from build123d import *

# Parameters (mm, degrees)
CROQUIS1_R                   = 3
CROQUIS1_R_2                 = 2
SALIENTE_EXTRUIR1_DEPTH      = 3.9
SALIENTE_EXTRUIR2_DEPTH      = 3.9
SALIENTE_EXTRUIR2_DEPTH_BACK = 3.9
REDONDEO1_R                  = 5
CROQUIS4_W                   = 2
CROQUIS4_H                   = 2
CORTAR_EXTRUIR1_DEPTH        = 46.769422107
CROQUIS5_R                   = 3.25
CORTAR_EXTRUIR2_DEPTH        = 46.769422107
REDONDEO3_R                  = 1


with BuildPart() as part:
    # Croquis1 → Saliente-Extruir1 (new body)
    with BuildSketch(Plane(origin=(0, 0, 0), x_dir=(1, 0, 0), z_dir=(0, 1, 0))):
        with Locations(Location((0, 0, 0), (0, 0, 270))):
            Circle(CROQUIS1_R)
        with Locations(Location((0, 0, 0), (0, 0, 270))):
            Circle(CROQUIS1_R_2, mode=Mode.SUBTRACT)
    extrude(amount=SALIENTE_EXTRUIR1_DEPTH)

    # Croquis3 → Saliente-Extruir2 (add, two sides: drawn at the far end of the back side and taken through both)
    with BuildSketch(Plane.XZ.offset(-SALIENTE_EXTRUIR2_DEPTH_BACK)):
        with BuildLine():
            Line((45, 3), (0, 3))
            ThreePointArc((0, 3), (2.121320344, 2.121320344), (3, 0))
            Line((3, 0), (45, 0))
            Line((45, 0), (45, 3))
        make_face()
    extrude(amount=SALIENTE_EXTRUIR2_DEPTH + SALIENTE_EXTRUIR2_DEPTH_BACK)

    # Redondeo1
    # the kernel refuses this fillet: 5 mm, written as the material it takes off along each edge
    with BuildSketch(Plane(origin=(45, 15.356439237, 0), x_dir=(-1, 0, 0), z_dir=(0, -1, 0))) as redondeo1_piece_1:
        with BuildLine():
            CenterArc((4.582575695, -5), REDONDEO1_R, 90, 66.421821522)
            Line((0, -3), (-0.091651514, -2.96))
            ThreePointArc((-0.091651514, -2.96), (-0.1, -1.5), (-0.1, 0))
            Line((-0.1, 0), (0, 0.1))
            Line((0, 0.1), (4.582575695, 0.1))
            Line((4.582575695, 0.1), (4.582575695, 0))
        make_face()
    extrude(amount=30.712878475, mode=Mode.SUBTRACT)

    # Croquis4 → Cortar-Extruir1 (cut, through all)
    with BuildSketch(Plane.XZ.offset(3.9)):
        with Locations((16, 3)):
            Rectangle(CROQUIS4_W, CROQUIS4_H)
    extrude(amount=-CORTAR_EXTRUIR1_DEPTH, mode=Mode.SUBTRACT)

    # Croquis5 → Cortar-Extruir2 (cut, through all)
    with BuildSketch(Plane.XZ.offset(3.9)):
        with Locations((33, -1.5)):
            Circle(CROQUIS5_R)
    extrude(amount=-CORTAR_EXTRUIR2_DEPTH, mode=Mode.SUBTRACT)

    # Redondeo3
    redondeo3_edges = [part.edges().sort_by_distance(p)[0] for p in [
        (30.116859351, 0, 0),
    ]]
    fillet(redondeo3_edges, radius=REDONDEO3_R)


solid = part.part
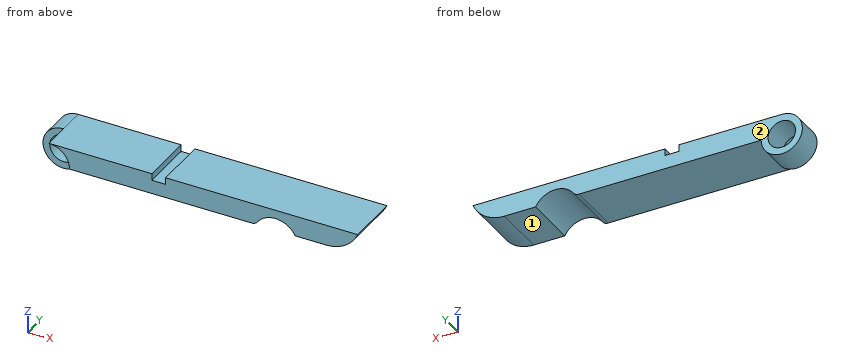
Geometry check sheet. Reference: the model listing, model coordinates, mm. Face numbers are marked on the shaded views. A direction names the side the tool comes from. Give positions to 0.01 mm unless a question says otherwise; leave off trailing zeros. Write each loop counter-clockwise with the first axis right and the second up, starting at its lowest first coordinate (ties: lowest second). Pieces come first, ordered by that corner, then holes. Notation, with made-up numbers: M 0.5,-5.75 L 37.5,-5.75 A10 ccw 37.5,7.25 Z; hole C -25.75,26 d3. An arc over 180 degrees is marked long. One line per question, with ' | ' between items.
1. Cross-section at D-D (x = 28.5). Enter the section's corners in (y, z).
Ans:
outline: M -3.9,0 L 3.9,0 L 3.9,3 L -3.9,3 Z
2. Cross-section at A-A (y = 1.25). Enter the section's corners in (x, z), plus the area to 3 significant figures.
Ans:
outline: M 0,3 A3 ccw long 3,0 L 29.56,0 A1 ccw 30.37,0.41 A3.25 cw 35.88,0 L 40.42,0 A5 ccw 45,3 L 17,3 L 17,2 L 15,2 L 15,3 Z; hole C 0,0 d4 | area: 131 mm2
3. Cross-section at C-C (y = -1.75). Enter the section's corners in (x, z).
Ans:
outline: M 0,3 A3 cw 3,0 L 29.56,0 A1 ccw 30.37,0.41 A3.25 cw 35.88,0 L 40.42,0 A5 ccw 45,3 L 17,3 L 17,2 L 15,2 L 15,3 Z
4. Scan lines: line 1 along Z through (x, y) = (24, 2); line 2 along Y through (x, z) = (2, 1.75); line 3 along X through (y, z) = (-2, 0.5). Record each from-to range of solid material in increasing order. Write a range as from..to.
Ans:
line 1: 0..3 | line 2: 0..3.9 | line 3: 2.96..30.44, 35.56..42.6
5. Gauge pin test, flat ends, axial feed: pin 1 (1.4 mm diameter, centred on x = 38, y = 0, fed in from -Z); pin 2 (0.5 mm diameter, centred on y = -0.5, z = 2.5, fed in from +X); pin 3 (1 mm diameter, centred on x = 35, y = -2, fed in from -Z). Record the tip position at first contact, or that the pin passes through.
Ans:
pin 1: z = 0 | pin 2: x = 44.88 | pin 3: z = 0.58
6. Cross-section at B-B (z = 1.25). Enter the section's corners in (x, y), plus the area to 3 significant figures.
Ans:
outline: M -2.73,0 L -1.56,0 L -1.56,3.9 L -2.73,3.9 Z; M 1.56,0 L 2.73,0 L 2.73,-3.9 L 31.27,-3.9 L 31.27,3.9 L 1.56,3.9 Z; M 34.73,-3.9 L 43.72,-3.9 L 43.72,3.9 L 34.73,3.9 Z | area: 302 mm2
7. Set-up check for the marked faces 1 and 2: record each of +Z, -Z, +X, -X, +Y, -Y from which the full face is reachable in a straight line by a thin tool's end or side.
Ans:
face 1: -Z, +X, +Y, -Y | face 2: +Z, -Z, +X, -X, +Y
